Part model, mm, in its own coordinate system. Face numbers are marked on the shaded views. A direction names the side the tool comes from. Round coordinates to 2 decimals unless told otherwise and drop trailing zeros. Loops run counter-clockwise (first coordinate to the right, second up) from the corner with the lowest first, then second, coordinate; pieces in that order, holes last. Notation, with made-up numbers: (-35.75, 15.25) -> (23.25, 15.25) arc R22 cw to (23.25, 38.25) -> close; hole circle Ø11 at (7, -17.5). An arc over 180 degrees is marked (long way). Answer as CSV lines item,"result".
Autodesk Inventor part; units mm, degrees
ref_plane "XZ Plane" through (0, 0, 0) normal (0, 1, 0) x (-1, 0, 0)
ref_plane "XY Plane" through (0, 0, 0) normal (0, 0, 1) x (1, 0, 0)
sketch "Sketch1" plane through (0, 0, 0) normal (0, 0, 1) x (1, 0, 0)
  circle A0 centre (0, 0) radius 5
  dimension "d0" = 10
extrude "Extrusion1" add sketch "Sketch1" against normal blind 50
ref_plane "Work Plane1" through (0, 0, -50) normal (0, 0, -1) x (-1, 0, 0)
ref_plane "Work Plane3" through (0, 0, -50) normal (0.7071068, 0, 0.7071068) x (0, -1, 0)
ref_plane "Work Plane2" through (0, 0, -50) normal (1, 0, 0) x (0, 1, 0)
sketch "Sketch2" plane through (0, 0, -50) normal (0.7071068, 0, 0.7071068) x (0, -1, 0)
  ellipse E0 centre (0, 0) end of major axis (-5, 0) minor radius 3.5355
  circle A0 centre (0, 0) radius 5
  point P0 (0, -35.3553)
  dimension "d14" = 10
extrude "Extrusion2" add sketch "Sketch2" along normal blind 70
ref_plane "Work Plane4" through (49.4975, 0, -0.5025) normal (0, 0, -1) x (-1, 0, 0)
sketch "Sketch3" plane through (49.4975, 0, -0.5025) normal (0, 0, -1) x (-1, 0, 0)
  ellipse E0 centre (0, 0) end of major axis (0, 5) minor radius 3.5355
  circle A0 centre (0, 0) radius 5
  point P0 (49.4975, 0)
extrude "Extrusion3" add sketch "Sketch3" along normal blind 60
ref_plane "Work Plane5" through (0, 0, -50) normal (0.3826834, 0, 0.9238795) x (0, -1, 0)
sketch "Sketch4" plane through (0, 0, -50) normal (0.3826834, 0, 0.9238795) x (0, -1, 0)
  circle A0 centre (0, 0) radius 2.8545
  point P0 (0, -19.1342)
extrude "Extrusion4" add sketch "Sketch4" along normal blind 1
ref_plane "Work Plane8" through (49.4975, 0, -0.5025) normal (0.3826834, 0, 0.9238795) x (0, 1, 0)
sketch "Sketch5" plane through (49.4975, 0, -0.5025) normal (0.3826834, 0, 0.9238795) x (0, 1, 0)
  circle A0 centre (0, 0) radius 2.6859
  point P0 (0, 45.922)
extrude "Extrusion5" add sketch "Sketch5" against normal blind 1
ref_plane "Work Plane7" through (49.4975, 0, -35.0025) normal (0, 0, -1) x (-1, 0, 0)
sketch "Sketch6" plane through (49.4975, 0, -35.0025) normal (0, 0, -1) x (-1, 0, 0)
  ellipse E0 centre (0, 0) end of major axis (0, -2.6859) minor radius 2.4814
  line L0 (-2.1727, -1.2973) -> (2.1727, -1.2973)
  line L1 (2.1727, -1.2973) -> (2.1727, 1.2973)
  line L2 (2.1727, 1.2973) -> (-2.1727, 1.2973)
  line L3 (-2.1727, 1.2973) -> (-2.1727, -1.2973)
  line L4 (0, -5) -> (0, 5)
  line L5 (-2.1727, -1.2973) -> (2.1727, 1.2973) construction
  line L6 (2.1727, -1.2973) -> (-2.1727, 1.2973) construction
  point P0 (49.4975, 0)
  point P1 (0, 0)
extrude "Extrusion6" add sketch "Sketch6" along normal blind 1 contours L0 L4 L2 L1 | L3 L2 L4 L0
properties part number "00_Beam_Ocular_Detectoin"
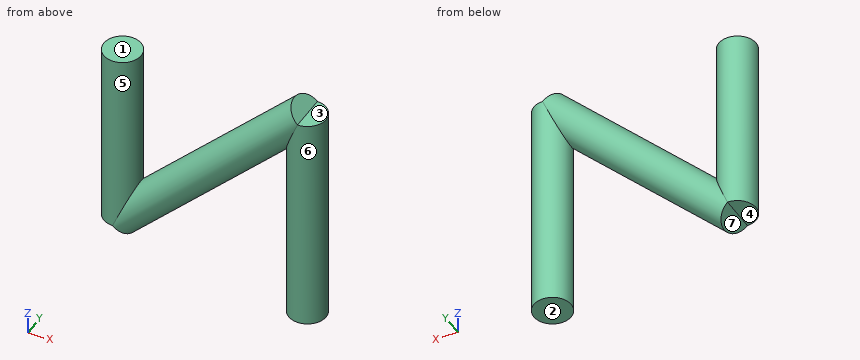
Q1. Drill centre lines: line 1 along X through (y, z) = (1.25, -29); line 2 along X through (y, z) = (-0.75, -34); line 3 along X through (y, z) = (-0.75, -6). Where is each one in solid material? Low to high.
Geometry results:
line 1,"-4.84 to 4.84, 14.15 to 27.85, 44.66 to 54.34"
line 2,"-4.94 to 4.94, 9.01 to 22.99, 44.55 to 54.44"
line 3,"-4.94 to 4.94, 37.01 to 54.44"
Q2. Which spindle directions (+Z, -Z, +X, -X, +Y, -Y) get a long thin tool onto all of the face, cutting with end or side? Do the marked faces 1, 2 and 3. Say none if no direction does.
Geometry results:
face 1,"+Z, -X, +Y, -Y"
face 2,"-Z, +X, -X, +Y, -Y"
face 3,"+Z, +X, +Y, -Y"
Q3. Saw through at C-C, the plane z = -21. Give the number of separate pieces and of enclosed holes in the cut face, then the cut area to 3 significant figures.
Geometry results:
separate pieces,"3"
enclosed holes,"0"
area,"268 mm2"
Q4. Drop flat-ended pins along their axis: P1, Ø2.5, axis at x = 52.5, y = 0.5, coming from the +Z side; P2, Ø4, axis at x = 42.5, z = -12, coming from the +Y side; P3, Ø1.5, axis at x = 3, z = -5.5, coming from the -Y side; P4, Ø10, axis at x = 36, z = -28.5, coming from the -Y side. Give the stop position or say it passes through.
Geometry results:
P1,"z = -0.5"
P2,"y = 4.86"
P3,"y = -4.47"
P4,"through"
Q5. Two-plate mould, pull along X, no slides. Class the marked faces 4, 5, 6 and 7: pulls with the +X half, pulls with the -X half, needs draft (parallel to the pull), parting line crosses it, or undercut.
Geometry results:
face 4,"needs draft"
face 5,"undercut"
face 6,"undercut"
face 7,"pulls with the -X half"
Q6. Saw through at A-A, the plane z = -57. Write the cut outline in (x, y).
Geometry results:
outline,"circle Ø10 at (49.5, 0)"
Q7. Saw through at B-B, the plane y = -1.75. Write the cut outline in (x, z), then the cut area to 3 significant figures.
Geometry results:
outline,"(-4.68, -50) -> (0, -50) -> (3.31, -53.31) -> (44.81, -11.81) -> (44.81, -60.5) -> (54.18, -60.5) -> (54.18, -0.5) -> (49.5, -0.5) -> (46.19, 2.81) -> (4.68, -38.69) -> (4.68, 0) -> (-4.68, 0) -> close"
area,"1,580 mm2"
